```python
from build123d import *

# Parameters (mm, degrees)
F0_W     = 5.842
F0_H     = 12.7
F0_R     = 3.175
F2_DEPTH = 25.4


with BuildPart() as f1:
    # F0 (on Front) → F1 (revolve)
    with BuildSketch(Plane.XZ):
        Polygon((5.842, 12.7), (5.842, 0), (66.294, 0), (66.294, 12.7), (56.134, 12.7), (56.134, 10.16), (10.16, 10.16), (10.16, 12.7), align=None)
        with Locations((2.921, 6.35)):
            Rectangle(F0_W, F0_H)
    revolve(axis=Axis((33.147, 0, 0), (-1, 0, 0)))

    # F0 (on Front) → F2 (join)
    with BuildSketch(Plane.XZ):
        Polygon((5.842, 12.7), (5.842, 0), (66.294, 0), (66.294, 12.7), (56.134, 12.7), (56.134, 10.16), (10.16, 10.16), (10.16, 12.7), align=None)
        with BuildLine():
            ThreePointArc((-8.1826630726, -5.5069827884), (-3.1957909266, -4.5493385486), (-0.9398, 0))
            ThreePointArc((-0.9398, 0), (-4.5919612295, 5.3297205562), (-10.8806298187, 3.8475430269))
            ThreePointArc((-10.8806298187, 3.8475430269), (-12.1459778134, -1.5837270034), (-8.1826630726, -5.5069827884))
        make_face()
        with Locations((-6.6548, 0)):
            Circle(F0_R, mode=Mode.SUBTRACT)
        with BuildLine():
            Line((-0.9398, 0), (0, 0))
            Line((0, 0), (0, 12.7))
            Line((0, 12.7), (5.842, 12.7))
            Line((5.842, 12.7), (5.842, 15.24))
            Line((5.842, 15.24), (-0.508, 15.24))
            Line((-0.508, 15.24), (-10.8806298187, 3.8475430269))
            ThreePointArc((-10.8806298187, 3.8475430269), (-4.5919612295, 5.3297205562), (-0.9398, 0))
        make_face()
        with Locations((2.921, 6.35)):
            Rectangle(F0_W, F0_H)
        with BuildLine():
            Line((5.842, 0), (0, 0))
            Line((0, 0), (-0.9398, 0))
            ThreePointArc((-0.9398, 0), (-3.1957909266, -4.5493385486), (-8.1826630726, -5.5069827884))
            Line((-8.1826630726, -5.5069827884), (5.842, -9.398))
            Line((5.842, -9.398), (5.842, 0))
        make_face()
        with Locations((-6.6548, 0)):
            Circle(F0_R)
    extrude(amount=F2_DEPTH)


solid = f1.part
```
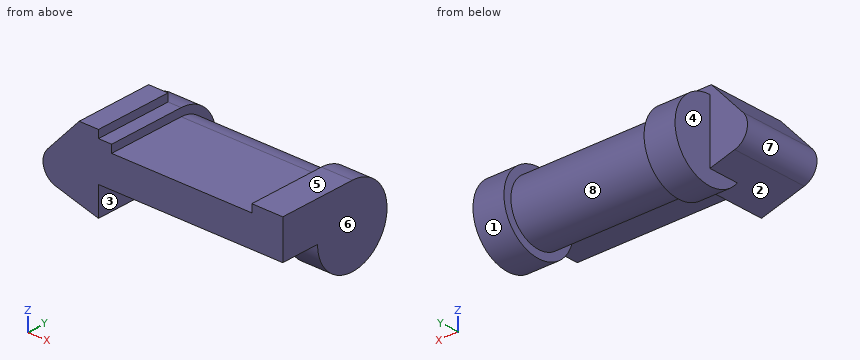
CAD build for the part. Positions are in the model's coordinates, mm. Face numbers are marked on the shaded views. A direction names the side the tool comes from. Round coordinates to 2 decimals unless told otherwise and drop trailing zeros. Write each loop counter-clockwise with the first axis right and the second up, starting at its lowest first coordinate (ties: lowest second). Pieces come first, ordered by that corner, then holes. Notation, with made-up numbers: (-34, 43.25) -> (-10, 43.25) arc R27 cw to (-10, 65.25) -> close; hole circle Ø7 at (50.25, 69.5). An arc over 180 degrees is marked (long way). Answer in a Markdown table with one row per item. Add a question column.
Item 1: Drop flat-ended pins along their axis: pin 1 Ø10 at (x, y) = (17, 3.5) entering from +Z; pin 2 Ø5 at (x, y) = (61, -6.5) entering from +Z; pin 3 Ø12 at (x, y) = (56, -7.5) entering from -Z; pin 4 Ø14.5 at (x, z) = (-3.5, 5) entering from +Y. Give the stop position or say it passes through.
Item 2: Which spindle directions (+Z, -Z, +X, -X, +Y, -Y) get a long thin tool onto all of the face, cutting with end or side? Do the marked faces 1, 2, 3, 4 and 5. Say none if no direction does.
Item 3: Saw through at A-A, the plane y = -15.5. Write the cut outline in (x, z) (3 decimals).
Item 4: Saw through at D-D, the plane z = 2.5. Write the cut outline in (x, y), then the cut area to 3 significant figures.
Item 5: Saw through at C-C, the plane x = 61. Write the cut outline in (y, z).
Item 6: Saw through at B-B, the plane z = -4.25. Write the cut outline in (x, y).
Item 7: Mould opens along X. For the marked faces 6, 7 and 8 say: pulls with the +X half, pulls with the -X half, needs draft (parallel to the pull), parting line crosses it, or undercut.
Item 8: Drill centre lines: line 1 (X direction, y = -6.5, z = -9.5); line 2 (Y direction, x = -8.5, z = 2.5); line 3 (X direction, y = 5.5, z = -5.25). Where is each one in solid material? Low to high. Write a range as from..to.
Findings below:
| question | item | result |
|---|---|---|
| 1 | pin 1 | stops at z = 10.16 |
| 1 | pin 2 | stops at z = 12.7 |
| 1 | pin 3 | stops at z = -12.61 |
| 1 | pin 4 | stops at y = 12.7 |
| 2 | face 1 | +X |
| 2 | face 2 | -Z, -X, -Y |
| 2 | face 3 | -Z, +X, -Y |
| 2 | face 4 | -Z, -X, +Y |
| 2 | face 5 | +Z, +X, +Y, -Y |
| 3 | outline | (-10.881, 3.848) arc R5.715 ccw to (-8.183, -5.507) -> (5.842, -9.398) -> (5.842, 0) -> (66.294, 0) -> (66.294, 12.7) -> (56.134, 12.7) -> (56.134, 10.16) -> (10.16, 10.16) -> (10.16, 12.7) -> (5.842, 12.7) -> (5.842, 15.24) -> (-0.508, 15.24) -> close |
| 4 | outline | (-11.79, -25.4) -> (66.29, -25.4) -> (66.29, 12.45) -> (56.13, 12.45) -> (56.13, 9.85) -> (10.16, 9.85) -> (10.16, 12.45) -> (0, 12.45) -> (0, 0) -> (-11.79, 0) -> close |
| 4 | area | 2,690 mm^2 |
| 5 | outline | (-25.4, 0) -> (-12.7, 0) arc R12.7 ccw (long way) to (0, 12.7) -> (-25.4, 12.7) -> close |
| 6 | outline | (-10.48, -25.4) -> (5.84, -25.4) -> (5.84, -11.97) -> (10.16, -11.97) -> (10.16, -9.23) -> (56.13, -9.23) -> (56.13, -11.97) -> (66.29, -11.97) -> (66.29, 11.97) -> (56.13, 11.97) -> (56.13, 9.23) -> (10.16, 9.23) -> (10.16, 11.97) -> (0, 11.97) -> (0, 0) -> (-10.48, 0) -> close |
| 7 | face 6 | pulls with the +X half |
| 7 | face 7 | pulls with the -X half |
| 7 | face 8 | undercut |
| 8 | line 1 | x = 0..10.16, 56.13..66.29 |
| 8 | line 2 | y = -25.4..0 |
| 8 | line 3 | x = 0..66.29 |
